Autodesk Inventor part; units mm, degrees
ref_plane "YZ Plane" through (0, 0, 0) normal (1, 0, 0) x (0, 1, 0)
ref_plane "XZ Plane" through (0, 0, 0) normal (0, 1, 0) x (-1, 0, 0)
ref_plane "XY Plane" through (0, 0, 0) normal (0, 0, 1) x (1, 0, 0)
sketch "Szkic1" plane through (0, 0, 0) normal (0, 1, 0) x (-1, 0, 0)
  circle A0 centre (0, 0) radius 10
  line L0 (27, 0) -> (27, -27)
  line L1 (27, -27) -> (0, -27)
  line L2 (27, 0) -> (27, 27)
  line L3 (27, 27) -> (0, 27)
  line L4 (-27, 0) -> (-27, -27)
  line L5 (-27, -27) -> (0, -27)
  line L6 (-27, 0) -> (-27, 27)
  line L7 (-27, 27) -> (0, 27)
  circle A1 centre (0, 0) radius 17.5
  dimension "d0" = 20
  dimension "d6" = 54
  dimension "d7" = 54
  dimension "d8" = 35
extrude "Wyciągnięcie proste1" add sketch "Szkic1" along normal blind 5
extrude "Wyciągnięcie proste2" add sketch "Szkic1" along normal blind 30 contours A1
properties part number "kapek"
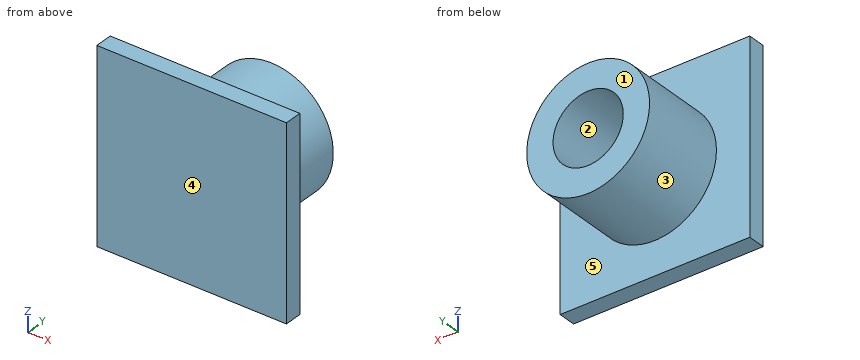
Here's how the part is built. I have some questions about the finished solid (model axes, mm). Face numbers are marked on the shaded views. A direction names the side the tool comes from. Coordinates: 2 decimals unless noted, no trailing zeros. Order: outer loops, then holes, each group sorted by start corner. A loop starts at its lowest first (then second) coordinate and runs counter-clockwise, first axis right, second up.
Item 1: If we mould it in two halves opening along X, with no side actions, what happens to the marked faces 1, 2 and 3? For each: +X half, -X half, draft (parallel to the pull), parting line (faces both ways), or undercut.
Result sheet:
face 1: draft
face 2: undercut
face 3: parting line
Item 2: If we section it at B-B on z = 14: List the corners of the cut face in (x, y) for me, plus the area to 3 significant figures.
Result sheet:
outline: (-27, 0) - (27, 0) - (27, 5) - (10.5, 5) - (10.5, 30) - (-10.5, 30) - (-10.5, 5) - (-27, 5) - close
area: 795 mm2
Item 3: If we section it at C-C on y = 9: List the corners of the cut face in (x, z) for me, plus the area to 3 significant figures.
Result sheet:
outline: circle Ø35 at (0, 0); hole circle Ø20 at (0, 0)
area: 648 mm2
Item 4: For P1, Ø1, axis at x = -5.5, z = 18, coming from the +Y side; P2, Ø4, axis at y = 17.5, z = 6.5, coming from the -X side; P3, Ø1.5, axis at y = 9, z = -5, coming from the +X side, each with a flat end and sliding along its axis, tell me the tip position at first contact or that it passes through.
Result sheet:
P1: stops at y = 5
P2: stops at x = -16.91
P3: stops at x = 16.98
Item 5: For the marked faces 4 and 5, which set-ups out of +Z, -Z, +X, -X, +Y, -Y let a thin tool reach every point of the face, with its end or its side?
Result sheet:
face 4: +Z, -Z, +X, -X, -Y
face 5: +Y
Item 6: I need wall thicknesses on line 1 (Z direction, x = 0, y = 11.25); line 2 (Y direction, x = 23, z = -5); line 3 (X direction, y = 23.5, z = -2). Which ranges of each line are inside material? Lowest first, please.
Result sheet:
line 1: z = -17.5 to -10, 10 to 17.5
line 2: y = 0 to 5
line 3: x = -17.39 to -9.8, 9.8 to 17.39
Item 7: If we section it at D-D on x = -14: List the corners of the cut face in (y, z) for me, plus the area to 3 significant figures.
Result sheet:
outline: (0, -27) - (5, -27) - (5, -10.5) - (30, -10.5) - (30, 10.5) - (5, 10.5) - (5, 27) - (0, 27) - close
area: 795 mm2
Item 8: If we section it at A-A on x = 0: List the corners of the cut face in (y, z) for me, plus the area to 3 significant figures.
Result sheet:
outline: (0, -27) - (5, -27) - (5, -17.5) - (30, -17.5) - (30, -10) - (5, -10) - (5, 10) - (30, 10) - (30, 17.5) - (5, 17.5) - (5, 27) - (0, 27) - close
area: 645 mm2
